Can you work these out from the drawing? Everything is in mm from the part's minimum corner. A direction names the side the tool comes from. Coordinates: 2 decimals unless noted, no trailing zeros. Loops run counter-clockwise (first coordinate to the right, second up) from the corner with the lowest first, then second, coordinate; pieces in that order, holes last. Notation, with made-up numbers: (59, -0.75) -> (72, -0.75) arc R15 ccw to (72, 25.25) -> close; hole circle Ø6 at (-34.5, 88). An arc over 180 degrees is marked (long way). Use one line per item in the form item = value. Start each with the question number.
(1) Imagine slicing it at C-C (x = 20). List the corners of the cut face in (y, z) for me.
(2) Imagine slicing it at B-B (x = 14). List the corners of the cut face in (y, z) for me.
(3) Imagine slicing it at A-A (y = 1.75). List the corners of the cut face in (x, z) for me.
(4) Imagine slicing it at D-D (y = 19.5). List the corners of the cut face in (x, z) for me, plus the area to 4 significant figures.
(5) I'm going to push flat-ended pins straight in: pin 1 (11 mm diameter, centred on x = 24.5, y = 11, fed in from -Z); pin 2 (3 mm diameter, centred on x = 3.5, z = 2.5, fed in from -Y). Where does each tip first touch, or does it pass through?
(6) I need wall thicknesses on line 1 (Z direction, x = 3.5, y = 4.5); line 2 (X direction, y = 3.25, z = 6); line 3 (X direction, y = 5.25, z = 2.5). Which ranges of each line are inside material? Lowest first, please. Write a range as [from, to].
(7) On a 3-axis mill with a long thin cutter (end or side, diameter ignored), from which of +Z, -Z, +X, -X, +Y, -Y can I reach the whole of each face in a straight line? I mean the marked faces 4 and 5. Say none if no direction works.
(8) Thinking about a two-plate mould opening in X: for the marked faces 1, 2 and 3, which applies, released by +X, released by -X, zero draft, split by the parting line, or undercut?
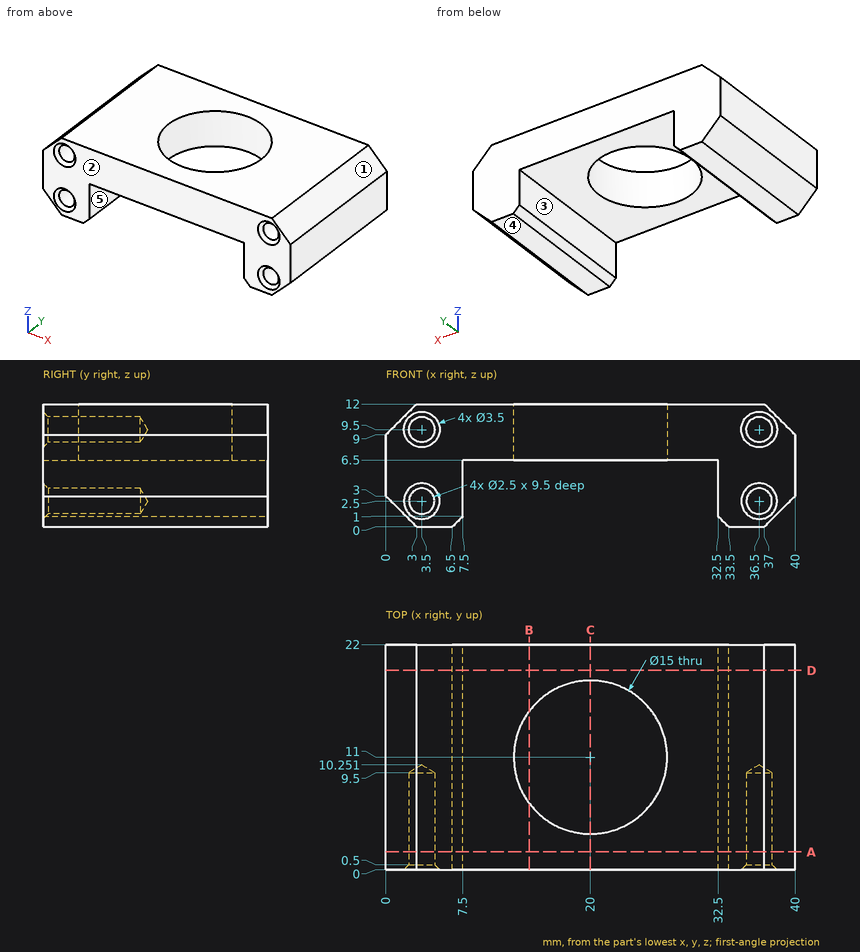
Worked out:
q1.outline = (0, 6.5) -> (3.5, 6.5) -> (3.5, 12) -> (0, 12) -> close; (18.5, 6.5) -> (22, 6.5) -> (22, 12) -> (18.5, 12) -> close
q2.outline = (0, 6.5) -> (6.5, 6.5) -> (6.5, 12) -> (0, 12) -> close; (15.5, 6.5) -> (22, 6.5) -> (22, 12) -> (15.5, 12) -> close
q3.outline = (0, 3) -> (3, 0) -> (6.5, 0) -> (7.5, 1) -> (7.5, 6.5) -> (32.5, 6.5) -> (32.5, 1) -> (33.5, 0) -> (37, 0) -> (40, 3) -> (40, 9) -> (37, 12) -> (3, 12) -> (0, 9) -> close; hole circle Ø2.5 at (3.5, 2.5); hole circle Ø2.5 at (3.5, 9.5); hole circle Ø2.5 at (36.5, 2.5); hole circle Ø2.5 at (36.5, 9.5)
q4.outline = (0, 3) -> (3, 0) -> (6.5, 0) -> (7.5, 1) -> (7.5, 6.5) -> (32.5, 6.5) -> (32.5, 1) -> (33.5, 0) -> (37, 0) -> (40, 3) -> (40, 9) -> (37, 12) -> (3, 12) -> (0, 9) -> close
q4.area = 298.5 mm2
q5.pin_1 = 6.5
q5.pin_2 = 0.25
q6.line_1 = [0, 1.25], [3.75, 8.25], [10.75, 12]
q6.line_2 = [0, 7.5], [32.5, 40]
q6.line_3 = [0.5, 2.25], [4.75, 7.5], [32.5, 35.25], [37.75, 39.5]
q7.face_4 = -Z, +X, -X, +Y, -Y
q7.face_5 = -Z, +Y, -Y
q8.face_1 = released by +X
q8.face_2 = zero draft
q8.face_3 = undercut
